Autodesk Inventor part; units mm, degrees
ref_plane "YZ Plane" through (0, 0, 0) normal (1, 0, 0) x (0, 1, 0)
ref_plane "XZ Plane" through (0, 0, 0) normal (0, 1, 0) x (-1, 0, 0)
ref_plane "XY Plane" through (0, 0, 0) normal (0, 0, 1) x (1, 0, 0)
sketch "Sketch1" plane through (0, 0, 0) normal (0, 0, 1) x (1, 0, 0)
  line L0 (-10, 5) -> (10, 5)
  line L1 (10, 5) -> (10, -5)
  line L2 (10, -5) -> (-10, -5)
  line L3 (-10, -5) -> (-10, 5)
  point P0 (0, 0)
  dimension "d0" = 20
  dimension "d1" = 10
  dimension "d2" = 10
  dimension "d3" = 5
extrude "Extrusion1" add sketch "Sketch1" along normal blind 6.1
sketch "Sketch2" plane through (0, 0, 6.1) normal (0, 0, 1) x (1, 0, 0)
  line L0 (10, 5) -> (-10, 5)
  line L1 (-1, 5) -> (0, 4)
  line L2 (0, 4) -> (10, 4)
  line L3 (10, -5) -> (10, 5)
  line L4 (10, 5) -> (10, 4)
  line L5 (-1, 5) -> (10, 5)
  point P0 (0, 0)
  dimension "d6" = 10
  dimension "d7" = 1
  dimension "d8" = 1
extrude "Extrusion2" cut sketch "Sketch2" against normal through all
sketch "Sketch3" plane through (0, 0, 6.1) normal (0, 0, 1) x (1, 0, 0)
  line L0 (-10, 5) -> (-10, -5)
  line L1 (10, -5) -> (10, 4)
  line L2 (-10, -5) -> (10, -5)
  point P0 (0, 0)
  point P1 (-4.75, -3)
  point P2 (4.75, -3)
  dimension "d36" = 5.25
  dimension "d38" = 2
  dimension "d39" = 2
  dimension "d41" = 9.5
sketch "Sketch4" plane through (0, 0, 6.1) normal (0, 0, 1) x (1, 0, 0)
  line L0 (-10, -5) -> (10, -5)
  line L1 (-10, 5) -> (-10, -5)
  line L2 (-6.75, -5) -> (-6.5, -5.5)
  line L3 (-6.5, -5.5) -> (-3, -5.5)
  line L4 (-3, -5.5) -> (-2.75, -5)
  line L5 (-6.75, -5) -> (-2.75, -5)
  line L6 (2.75, -5) -> (3, -5.5)
  line L7 (3, -5.5) -> (6.5, -5.5)
  line L8 (6.5, -5.5) -> (6.75, -5)
  line L9 (2.75, -5) -> (6.75, -5)
  line L10 (10, -5) -> (10, 4)
  point P0 (0, 0)
  point P1 (6.75, -5)
  dimension "d16" = 0.5
  dimension "d17" = 4
  dimension "d19" = 3.5
  dimension "d20" = 0.25
  dimension "d22" = 4
  dimension "d23" = 3.5
  dimension "d24" = 0.25
  dimension "d25" = 0.5
  dimension "d26" = 0
  dimension "d40" = 3.5
  dimension "d43" = 3.5
extrude "Extrusion3" add sketch "Sketch4" against normal blind 6.1
hole "Hole1" at (-4.75, -3, 6.1) at (4.75, -3, 6.1) direction (0, 0, -1) diameter 2.6 end through all
sketch "Sketch5" plane through (-2.75, -5, 0) normal (0, -1, 0) x (1, 0, 0)
  line L0 (-7.25, 0) -> (-7.25, 6.1)
  line L1 (-7.25, 3.05) -> (12.75, 3.05)
  line L2 (12.75, 0) -> (12.75, 6.1)
  line L3 (-5.15, 1.45) -> (-5.75, 1.45)
  line L4 (-5.75, 1.45) -> (-5.75, 4.65)
  line L5 (-5.75, 4.65) -> (-5.15, 4.65)
  line L6 (-5.15, 4.65) -> (-5.15, 1.45)
  line L7 (-5.15, 1.45) -> (-5.75, 4.65) construction
  line L8 (-5.75, 1.45) -> (-5.15, 4.65) construction
  line L9 (3.95, 1.45) -> (3.35, 1.45)
  line L10 (3.35, 1.45) -> (3.35, 4.65)
  line L11 (3.35, 4.65) -> (3.95, 4.65)
  line L12 (3.95, 4.65) -> (3.95, 1.45)
  line L13 (3.95, 1.45) -> (3.35, 4.65) construction
  line L14 (3.35, 1.45) -> (3.95, 4.65) construction
  line L15 (11.25, 1.45) -> (10.65, 1.45)
  line L16 (10.65, 1.45) -> (10.65, 4.65)
  line L17 (10.65, 4.65) -> (11.25, 4.65)
  line L18 (11.25, 4.65) -> (11.25, 1.45)
  line L19 (11.25, 1.45) -> (10.65, 4.65) construction
  line L20 (10.65, 1.45) -> (11.25, 4.65) construction
  point P0 (2.75, 0)
  point P1 (-5.45, 3.05)
  point P2 (3.65, 3.05)
  point P3 (10.95, 3.05)
  dimension "d44" = 3.2
  dimension "d45" = 0.6
  dimension "d46" = 0.6
  dimension "d47" = 0.6
  dimension "d48" = 1.5
  dimension "d49" = 1.5
  dimension "d50" = 8.5
extrude "Extrusion4" add sketch "Sketch5" along normal blind 4.5
chamfer "Chamfer1" distance 0.5 angle 45 6 edges at (-8.2, -9.5, 4.65) (-8.2, -9.5, 1.45) (0.9, -9.5, 4.65) (0.9, -9.5, 1.45) (8.2, -9.5, 4.65) (8.2, -9.5, 1.45)
sketch "Sketch6" plane through (8.5, -5, 4.65) normal (1, 0, 0) x (0, 0, -1)
  line L0 (3.2, 0) -> (3.2, -4)
  line L1 (2.7, -4.5) -> (0.5, -4.5)
  point P0 (4.65, 5)
  point P1 (1.6, -2.9)
  dimension "d56" = 1.6
  dimension "d57" = 1.6
hole "Hole2" at (8.5, -7.9, 3.05) direction (-1, 0, 0) diameter 1.5 end through all
sketch "Sketch7" plane through (0, 0, 6.1) normal (0, 0, 1) x (1, 0, 0)
  line L0 (-10, 5) -> (-10, -5)
  line L1 (-1, 5) -> (-10, 5)
  point P0 (0, 0)
  point P1 (-7, 3.5)
  dimension "d65" = 3
  dimension "d66" = 1.5
hole "Hole3" at (-7, 3.5, 6.1) direction (0, 0, -1) diameter 1 end through all
Geometry check sheet. Reference: the model listing, model coordinates, mm. A direction names the side the tool comes from. Coordinates: 2 decimals unless noted, no trailing zeros. Write each loop counter-clockwise with the first axis right and the second up, starting at its lowest first coordinate (ties: lowest second). Pieces come first, ordered by that corner, then holes. Notation, with made-up numbers: (48.5, 15.5) -> (55.5, 15.5) arc R14 ccw to (55.5, 37.5) -> close; hole circle Ø3 at (12, 71.25). An arc over 180 degrees is marked (long way). One line per question, with ' | ' between items.
1. Draft check along Y on faces 6 (the flat face through (5, -5.5, 3)), 7 (the flat face through (-8.5, -7, 3)), 8 (the cylindrical face through (-7, 4, 3)). Enter one of: +Y half, -Y half, draft (parallel to the pull), parting line (faces both ways), or undercut.
Answers:
face 6: -Y half | face 7: draft | face 8: undercut
2. Depth check by flat-ended pin: pin 1 Ø3.5 at (x, y) = (4.75, -3) entering from +Z; pin 2 Ø0.7 at (x, y) = (1, -7.5) entering from -Z; pin 3 Ø1.6 at (y, z) = (-7.5, 3.5) entering from -X; pin 4 Ø1.5 at (x, z) = (6, 4.5) entering from -Y. Enter the tip coordinate at first touch or a pass-through.
Answers:
pin 1: stops at z = 6.1 | pin 2: stops at z = 1.45 | pin 3: stops at x = -8.5 | pin 4: stops at y = -5.5
3. Cross-section at D-D on y = -6. Record the cut outline in (x, z), and give its area (3 significant figures).
Answers:
outline: (-8.5, 1.45) -> (-7.9, 1.45) -> (-7.9, 4.65) -> (-8.5, 4.65) -> close; (0.6, 1.45) -> (1.2, 1.45) -> (1.2, 4.65) -> (0.6, 4.65) -> close; (7.9, 1.45) -> (8.5, 1.45) -> (8.5, 4.65) -> (7.9, 4.65) -> close | area: 5.76 mm²
4. Cross-section at B-B on x = 4.75. Record the cut outline in (y, z), and give its area (3 significant figures).
Answers:
outline: (-5.5, 0) -> (-4.3, 0) -> (-4.3, 6.1) -> (-5.5, 6.1) -> close; (-1.7, 0) -> (4, 0) -> (4, 6.1) -> (-1.7, 6.1) -> close | area: 42.1 mm²
5. Set-up check for faces 1 (the flat face through (8.5, -7, 3)), 2 (the flat face through (-7.9, -7, 3)), 3 (the flat face through (-10, 0, 3)), 4 (the flat face through (5, 4, 3)), 5 (the flat face through (0, 0, 6.1)): record each of +Z, -Z, +X, -X, +Y, -Y from which the full face is reachable in a straight line by a thin tool's end or side.
Answers:
face 1: +Z, -Z, +X, -Y | face 2: +Z, -Z, -Y | face 3: +Z, -Z, -X, +Y, -Y | face 4: +Z, -Z, +X, +Y | face 5: +Z, +X, -X, +Y, -Y
6. Thickness scan on probe 1 along X at (y, z) = (-3, 2); probe 2 along Y at (x, z) = (-8.2, 3.05); probe 3 along Y at (x, z) = (-4.75, 3.25). Record the ranges inside material, lowest first. Write a range as from..to.
Answers:
probe 1: x = -10..-6.05, -3.45..3.45, 6.05..10 | probe 2: y = -9.5..-8.65, -7.15..5 | probe 3: y = -5.5..-4.3, -1.7..5
7. Cross-section at A-A on y = -3. Record the cut outline in (x, z).
Answers:
outline: (-10, 0) -> (-6.05, 0) -> (-6.05, 6.1) -> (-10, 6.1) -> close; (-3.45, 0) -> (3.45, 0) -> (3.45, 6.1) -> (-3.45, 6.1) -> close; (6.05, 0) -> (10, 0) -> (10, 6.1) -> (6.05, 6.1) -> close
8. Cross-section at C-C on y = 3.5. Record the cut outline in (x, z), and give its area (3 significant figures).
Answers:
outline: (-10, 0) -> (-7.5, 0) -> (-7.5, 6.1) -> (-10, 6.1) -> close; (-6.5, 0) -> (10, 0) -> (10, 6.1) -> (-6.5, 6.1) -> close | area: 116 mm²
